Check sheet for the modelled part. Datum: model origin and axes. Units: mm. Face numbers are marked on the shaded views. Round coordinates to 2 decimals unless told otherwise and drop trailing zeros. One line per item, written item: value.
from build123d import *

# Parameters (mm, degrees)
SKETCH4_W               = 141.009584828
SKETCH4_H               = 12
CUT_EXTRUDE1_DEPTH      = 53.911904977
CUT_EXTRUDE1_DEPTH_BACK = 53.911904977
CUT_EXTRUDE2_DEPTH      = 20


with BuildPart() as part:
    # Sketch3 → Revolve2 (revolve)
    with BuildSketch(Plane.XY):
        with BuildLine():
            Line((0, 0), (0, 60.774821803))
            ThreePointArc((0, 60.774821803), (17.600685917, 22.677819891), (52.911904877, 0))
            Line((52.911904877, 0), (0, 0))
        make_face()
    revolve(axis=Axis((0, 0, 0), (0, 1, 0)))

    # Sketch4 → Cut-Extrude1 (cut, two sides)
    with BuildSketch(Plane(origin=(0, 0, 0), x_dir=(0, 0, -1), z_dir=(1, 0, 0))) as cut_extrude1_sk:
        with Locations((0, 6)):
            Rectangle(SKETCH4_W, SKETCH4_H)
    extrude(amount=CUT_EXTRUDE1_DEPTH, mode=Mode.SUBTRACT)
    extrude(cut_extrude1_sk.sketch, amount=-CUT_EXTRUDE1_DEPTH_BACK, mode=Mode.SUBTRACT)

    # Sketch5 → Cut-Extrude2 (cut)
    with BuildSketch(Plane.XZ.offset(-12)):
        Polygon((-5.41643054, 4.942227588), (-6.988309913, -2.219652652), (-1.571879373, -7.16188024), (5.41643054, -4.942227588), (6.988309913, 2.219652652), (1.571879373, 7.16188024), align=None)
    extrude(amount=-CUT_EXTRUDE2_DEPTH, mode=Mode.SUBTRACT)


solid = part.part
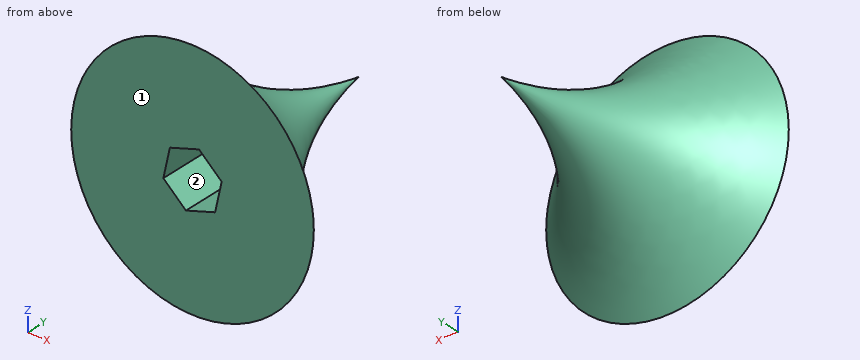
Q1. Draft check along Z on the marked faces 1 and 2. Enter one of: pulls with the +Z half, pulls with the -Z half, needs draft (parallel to the pull), parting line crosses it, or undercut.
Completed:
face 1: needs draft
face 2: undercut
Q2. Scan lines: line 1 (X direction, y = 42, z = 4); line 2 (Y direction, x = -11.5, z = -17.5); line 3 (Y direction, x = 5.5, z = 10.5). Record each from-to range of solid material in increasing order. Write a range as [from, to].
Completed:
line 1: [-3.62, 3.62]
line 2: [12, 19.09]
line 3: [12, 30.19]
Q3. Depth check by flat-ended pin: P1, Ø3, axis at x = -14, z = 8, coming from the +Y side; P2, Ø11, axis at x = 3.5, z = 0.5, coming from the -Y side; P3, Ø1, axis at y = 48, z = -2, coming from the +X side; P4, Ø10, axis at y = 17.5, z = -4.5, coming from the -X side. Enter the tip coordinate at first touch or a pass-through.
Completed:
P1: y = 26.32
P2: y = 12
P3: x = 2.76
P4: x = -28.09
